Here's how the part is built. I have some questions about the finished solid (model axes, mm). A direction names the side the tool comes from. Round coordinates to 2 decimals unless told otherwise and drop trailing zeros. Order: outer loops, then holes, each group sorted by start corner. A loop starts at its lowest first (then second) coordinate and runs counter-clockwise, first axis right, second up.
```python
from build123d import *

# Parameters (mm, degrees)
CUT_EXTRUDE1_DEPTH = 3


with BuildPart() as part:
    # Sketch1 → Revolve1 (revolve)
    with BuildSketch(Plane.XY, mode=Mode.PRIVATE) as revolve1_sk:
        with BuildLine():
            Line((0, -40), (1.6, -40))
            ThreePointArc((1.6, -40), (1.77941078, -39.713070248), (1.907878403, -39.4))
            Line((1.907878403, -39.4), (3, -38.307878403))
            Line((3, -38.307878403), (3, 0))
            Line((3, 0), (5, 0))
            Line((5, 0), (5, 6))
            Line((5, 6), (0, 6))
            Line((0, 6), (0, -40))
        make_face()
    revolve(revolve1_sk.sketch.rotate(Axis((0, 61.691642626, 0), (0, -1, 0)), 90), axis=Axis((0, 61.691642626, 0), (0, -1, 0)))

    # Sketch2 → Cut-Extrude1 (cut)
    with BuildSketch(Plane(origin=(0, 6, 0), x_dir=(-1, 0, 0), z_dir=(0, 1, 0))):
        Polygon((-1.443375673, -2.5), (1.443375673, -2.5), (2.886751346, 0), (1.443375673, 2.5), (-1.443375673, 2.5), (-2.886751346, 0), align=None)
    extrude(amount=-CUT_EXTRUDE1_DEPTH, mode=Mode.SUBTRACT)


solid = part.part
```
1. If we section it at D-D, the plane x = 4.25: Write out the boundary of the cut face in (y, z).
Evaluation:
outline: (0, -2.63) - (6, -2.63) - (6, 2.63) - (0, 2.63) - close
2. If we section it at C-C, the plane z = 4: Write out the boundary of the cut face in (x, y).
Evaluation:
outline: (-3, 0) - (3, 0) - (3, 6) - (-3, 6) - close
3. If we section it at B-B, the plane y = -36: Write out the boundary of the cut face in (x, z), and give its area (3 significant figures).
Evaluation:
outline: circle Ø6 at (0, 0)
area: 28.3 mm2
4. I'm going to push flat-ended pins straight in: P1, Ø2, axis at y = -31, z = -3, coming from the +X side; P2, Ø1.5, axis at x = -2.5, z = -3.5, coming from the -Y side; P3, Ø4, axis at x = -3, y = -35, coming from the +Z side. Where does each tip first touch, or does it pass through?
Evaluation:
P1: stops at x = 2.24
P2: stops at y = 0
P3: stops at z = 2.83
5. If we section it at A-A, the plane x = 0: Write out the boundary of the cut face in (y, z).
Evaluation:
outline: (-40, -1.6) arc R2 ccw to (-39.4, -1.91) - (-38.31, -3) - (0, -3) - (0, -5) - (6, -5) - (6, -2.5) - (3, -2.5) - (3, 2.5) - (6, 2.5) - (6, 5) - (0, 5) - (0, 3) - (-38.31, 3) - (-39.4, 1.91) arc R2 ccw to (-40, 1.6) - close
6. If we mould it in two halves opening along X, with no side actions, what happens to faces 1 (the flat face through (0, 5, -2.5)), 2 (the flat face through (0, -40, 0)), 3 (the cylindrical face through (-0.9, -18.89, 2.86))? For each: released by +X, released by -X, zero draft, split by the parting line, or undercut.
Evaluation:
face 1: undercut
face 2: zero draft
face 3: split by the parting line
7. On a 3-axis mill with a long thin cutter (end or side, diameter ignored), from which of +Z, -Z, +X, -X, +Y, -Y can I reach the whole of each face in a straight line? I mean faces 4 (the flat face through (3.3, 0, 0.1)), 5 (the flat face through (2, 6, 2)), 6 (the flat face through (0, 3, 0)). Say none if no direction works.
Evaluation:
face 4: -Y
face 5: +Z, -Z, +X, -X, +Y
face 6: +Y
8. I need wall thicknesses on probe 1 along Y at (x, z) = (0.5, 1); probe 2 along Y at (x, z) = (-4.25, 0.25); probe 3 along X at (y, z) = (-5.5, 1.25). Which ranges of each line are inside material? Lowest first, please.
Evaluation:
probe 1: y = -40 to 3
probe 2: y = 0 to 6
probe 3: x = -2.73 to 2.73
